```python
from build123d import *

# Parameters (mm, degrees)
SKETCH1_R                = 16.5
BOSS_EXTRUDE1_DEPTH      = 30
SKETCH2_R                = 2
BOSS_EXTRUDE2_DEPTH      = 2
SKETCH3_R                = 18.5
BOSS_EXTRUDE3_DEPTH      = 22
SKETCH5_R                = 6
BOSS_EXTRUDE4_DEPTH      = 6
SKETCH6_R                = 3
BOSS_EXTRUDE5_DEPTH      = 15
CUT_EXTRUDE1_START       = -12
CUT_EXTRUDE1_DEPTH       = 12
M3_CLEARANCE_HOLE1_D     = 3.4
M3_CLEARANCE_HOLE1_DEPTH = 10
M3_CLEARANCE_HOLE1_TIP   = 1.021463052
SKETCH16_R               = 17.3
BOSS_EXTRUDE6_DEPTH      = 15


with BuildPart() as part:
    # Sketch1 → Boss-Extrude1 (new body)
    with BuildSketch(Plane(origin=(0, 0, 0), x_dir=(1, 0, 0), z_dir=(0, 1, 0))):
        with Locations(Location((0, 0, 0), (0, 0, 270))):
            Circle(SKETCH1_R)
    extrude(amount=BOSS_EXTRUDE1_DEPTH)

    # Sketch2 → Boss-Extrude2 (add)
    with BuildSketch(Plane.XZ):
        with Locations(Location((0, 0, 0), (0, 0, 90))):
            Circle(SKETCH2_R)
    extrude(amount=BOSS_EXTRUDE2_DEPTH)

    # Sketch3 → Boss-Extrude3 (add)
    with BuildSketch(Plane(origin=(0, 30, 0), x_dir=(1, 0, 0), z_dir=(0, 1, 0))):
        with Locations(Location((0, 0, 0), (0, 0, 270))):
            Circle(SKETCH3_R)
    extrude(amount=BOSS_EXTRUDE3_DEPTH)

    # Sketch5 → Boss-Extrude4 (add)
    with BuildSketch(Plane(origin=(0, 52, 0), x_dir=(1, 0, 0), z_dir=(0, 1, 0))):
        with Locations(Location((7, 0, 0), (0, 0, 270))):
            Circle(SKETCH5_R)
    extrude(amount=BOSS_EXTRUDE4_DEPTH)

    # Sketch6 → Boss-Extrude5 (add)
    with BuildSketch(Plane(origin=(0, 58, 0), x_dir=(1, 0, 0), z_dir=(0, 1, 0))):
        with Locations(Location((7, 0, 0), (0, 0, 270))):
            Circle(SKETCH6_R)
    extrude(amount=BOSS_EXTRUDE5_DEPTH)

    # Sketch9 → Cut-Extrude1 (cut)
    with BuildSketch(Plane(origin=(0, 73, 0), x_dir=(1, 0, 0), z_dir=(0, 1, 0)).offset(CUT_EXTRUDE1_START)):
        with BuildLine():
            ThreePointArc((9.5, -1.658312395), (9.872281323, -0.866025404), (10, 0))
            Line((10, 0), (9.5, 0))
            Line((9.5, 0), (9.5, -1.658312395))
        make_face()
        with BuildLine():
            Line((9.5, 0), (10, 0))
            ThreePointArc((10, 0), (9.872281323, 0.866025404), (9.5, 1.658312395))
            Line((9.5, 1.658312395), (9.5, 0))
        make_face()
    extrude(amount=CUT_EXTRUDE1_DEPTH, mode=Mode.SUBTRACT)

    # M3 Clearance Hole1
    with Locations(Plane(origin=(0, 52, 0), x_dir=(1, 0, 0), z_dir=(0, 1, 0))):
        with Locations((0, -15.5), (-13.423393759, -7.75), (0, 15.5), (-13.423393759, 7.75), (13.423393759, -7.75), (13.423393759, 7.75)):
            Hole(M3_CLEARANCE_HOLE1_D / 2, depth=M3_CLEARANCE_HOLE1_DEPTH)
            with Locations((0, 0, -(M3_CLEARANCE_HOLE1_DEPTH + M3_CLEARANCE_HOLE1_TIP / 2))):  # 118° drill point
                Cone(0, M3_CLEARANCE_HOLE1_D / 2, M3_CLEARANCE_HOLE1_TIP, mode=Mode.SUBTRACT)

    # Sketch16 → Boss-Extrude6 (add)
    with BuildSketch(Plane.XZ):
        with Locations(Location((0, 0, 0), (0, 0, 270))):
            Circle(SKETCH16_R)
    extrude(amount=BOSS_EXTRUDE6_DEPTH)


solid = part.part
```
Check sheet for the modelled part. Datum: model origin and axes. Units: mm. A direction names the side the tool comes from. Give positions to 0.01 mm unless a question says otherwise; leave off trailing zeros. Write each loop counter-clockwise with the first axis right and the second up, starting at its lowest first coordinate (ties: lowest second). Pieces come first, ordered by that corner, then holes. Notation, with made-up numbers: (-26.75, -15.5) - (-21.75, -15.5) arc R16 ccw to (-21.75, -3.5) - close; hole circle Ø9 at (-22, 42). An arc over 180 degrees is marked (long way). Answer as a JSON object with one key per item and string values. Group by question number.
1) Release check for a two-part mould opening along Y. For faces 1 (the face through (-16.108, 14.79, -3.577)), 2 (the face through (0, -15, 0)), 3 (the face through (12.95, 54.96, -0.78)), 4 (the face through (-0.064, 41.156, -15.212)) record: pulls with the +Y half, pulls with the -Y half, needs draft (parallel to the pull), parting line crosses it, or undercut.
2) Sectioned sample at B-B (y = 63). Record the cut outline in (x, z).
3) Sectioned sample at D-D (z = 5). Record the cut outline in (x, y).
4) Access from +Z, -Z, +X, -X, +Y, -Y to the whole of each face (thin tool, end or side, straight path). Record for faces 5 (the face through (9.5, 67, 0)), 6 (the face through (0, 30, -17)), 7 (the face through (4.07, 65.4, -0.65)).
5) Depth check by flat-ended pin: P1, Ø2, axis at y = 32.5, z = -6.5, coming from the -X side; P2, Ø10, axis at x = -9.5, y = 32.5, coming from the +Z side; P3, Ø5, axis at y = 13.5, z = 11, coming from the +X side. Enter the tip coordinate at first touch or a pass-through.
6) Thickness scan on probe 1 along Y at (x, z) = (5.5, 16); probe 2 along X at (y, z) = (44, 7); probe 3 along Z at (x, y) = (0.5, 41.5). Record the ranges inside material, lowest first. Write a range as from..to.
7) Sectioned sample at A-A (z = 0). Record the cut outline in (x, y).
8) Sectioned sample at C-C (x = 7). Record the cut outline in (y, z).
Geometry results:
{
 "1": {"face 1": "undercut", "face 2": "pulls with the -Y half", "face 3": "needs draft", "face 4": "pulls with the +Y half"},
 "2": {"outline": "(9.5, -1.66) - (9.5, 1.66) arc R3 ccw (long way) to start"},
 "3": {"outline": "(-17.81, 30) - (-15.72, 30) - (-15.72, 0) - (-16.56, 0) - (-16.56, -15) - (16.56, -15) - (16.56, 0) - (15.72, 0) - (15.72, 30) - (17.81, 30) - (17.81, 52) - (10.32, 52) - (10.32, 58) - (3.68, 58) - (3.68, 52) - (-17.81, 52) - close"},
 "4": {"face 5": "+Z, -Z, +X, +Y", "face 6": "none", "face 7": "+Y"},
 "5": {"P1": "stops at x = -17.66", "P2": "stops at z = 17.94", "P3": "stops at x = 14.14"},
 "6": {"probe 1": "y = -15..0, 30..52", "probe 2": "x = -17.12..-14.95, -11.9..11.9, 14.95..17.12", "probe 3": "z = -18.49..-16.21, -14.79..14.79, 16.21..18.49"},
 "7": {"outline": "(-18.5, 30) - (-16.5, 30) - (-16.5, 0) - (-17.3, 0) - (-17.3, -15) - (17.3, -15) - (17.3, 0) - (16.5, 0) - (16.5, 30) - (18.5, 30) - (18.5, 52) - (13, 52) - (13, 58) - (10, 58) - (10, 61) - (9.5, 61) - (9.5, 73) - (4, 73) - (4, 58) - (1, 58) - (1, 52) - (-18.5, 52) - close"},
 "8": {"outline": "(-15, -15.82) - (0, -15.82) - (0, -14.94) - (30, -14.94) - (30, -17.12) - (52, -17.12) - (52, -6) - (58, -6) - (58, -3) - (73, -3) - (73, 3) - (58, 3) - (58, 6) - (52, 6) - (52, 17.12) - (30, 17.12) - (30, 14.94) - (0, 14.94) - (0, 15.82) - (-15, 15.82) - close"}
}
